Here's the drawing with two shaded views (mm, measured from the low corner). I have some questions. Give positions to 0.01 mm unless a question says otherwise; leave off trailing zeros. Write each loop counter-clockwise with the first axis right and the second up, starting at its lowest first coordinate (ties: lowest second). Pieces come first, ordered by that corner, then holes. Notation, with made-up numbers: (24.25, 3) -> (30.25, 3) arc R8 cw to (30.25, 16) -> close; hole circle Ø8 at (-9, 6). An arc over 180 degrees is marked (long way). Put each result on its own line as item: value. Start each with the question number.
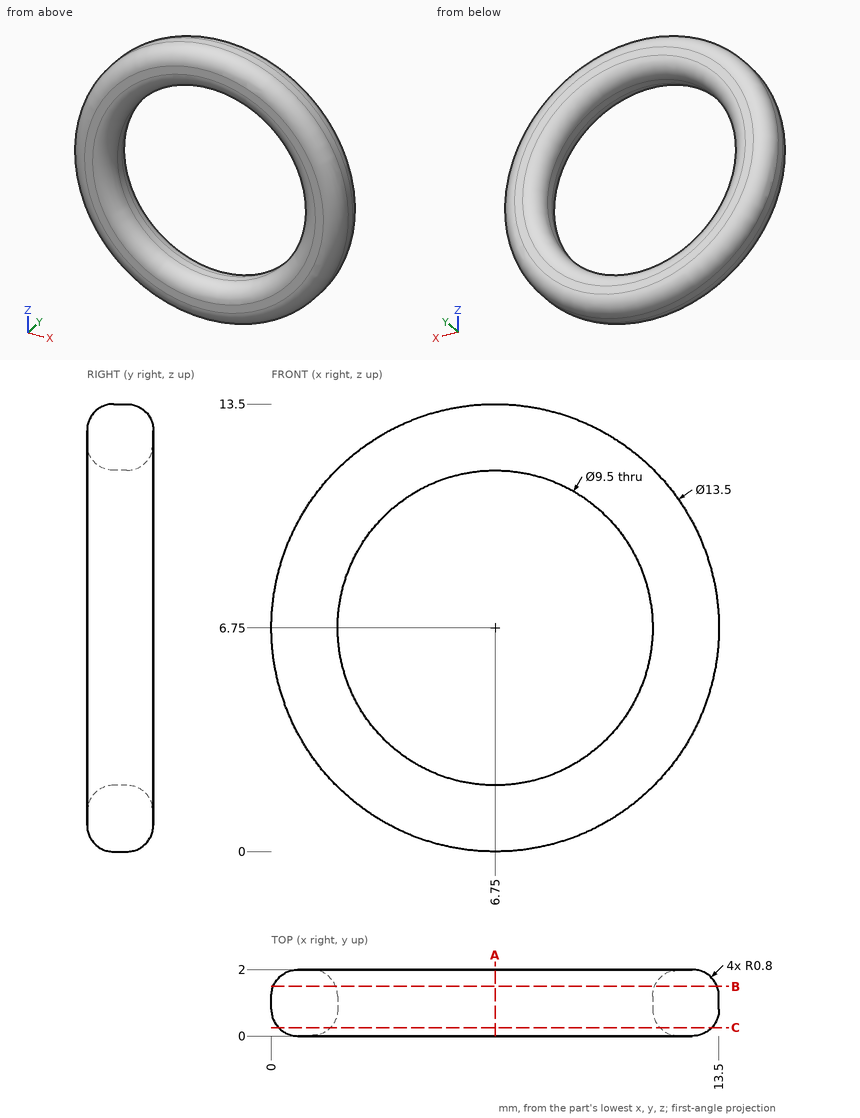
1) I want a section at A-A, the plane x = 6.75. Write out the boundary of the cut face in (y, z).
2) I want a section at C-C, the plane y = 0.25. Write out the boundary of the cut face in (x, z).
3) I need wall thicknesses on probe 1 along X at (y, z) = (1, 6.75); probe 2 along Y at (x, z) = (1, 8.5); probe 3 along Z at (x, y) = (10.5, 1.1). Which ranges of each line are inside material? Lowest first, please.
4) I want a section at B-B, the plane y = 1.5. Write out the boundary of the cut face in (x, z).
Established:
1. outline: (0, 0.8) arc R0.8 ccw to (0.8, 0) -> (1.2, 0) arc R0.8 ccw to (2, 0.8) -> (2, 1.2) arc R0.8 ccw to (1.2, 2) -> (0.8, 2) arc R0.8 ccw to (0, 1.2) -> close; (0, 12.3) arc R0.8 ccw to (0.8, 11.5) -> (1.2, 11.5) arc R0.8 ccw to (2, 12.3) -> (2, 12.7) arc R0.8 ccw to (1.2, 13.5) -> (0.8, 13.5) arc R0.8 ccw to (0, 12.7) -> close
2. outline: circle Ø13.06 at (6.75, 6.75); hole circle Ø9.94 at (6.75, 6.75)
3. probe 1: x = 0 to 2, 11.5 to 13.5
3. probe 2: y = 0 to 2
3. probe 3: z = 1.14 to 3.83, 9.67 to 12.36
4. outline: circle Ø13.38 at (6.75, 6.75); hole circle Ø9.62 at (6.75, 6.75)
